Part model, mm, in its own coordinate system. A direction names the side the tool comes from. Round coordinates to 2 decimals unless told otherwise and drop trailing zeros. Write each loop counter-clockwise with the first axis right and the second up, starting at its lowest first coordinate (ties: lowest second). Pieces come first, ordered by that corner, then holes. Notation, with made-up numbers: (19, 55) -> (34, 55) arc R24 cw to (34, 88) -> close; hole circle Ø1 at (85, 25). An arc over 180 degrees is marked (long way). Return JSON: item names as keys, results as strings. Group by question number.
(1) Tool access for faces 4 (the cylindrical face through (9.139, 14.334, 64.09)), 5 (the flat face through (0, 0, -10)), 6 (the flat face through (-5, -32, 120)): list every direction of +Z, -Z, +X, -X, +Y, -Y with a clear straight run to the whole face (end or side of a thin tool).
(2) Mould opens along X. For faces 1 (the flat face through (0, 0, 0)), 2 (the flat face through (15.4, 8.4, 130)), 3 (the cylindrical face through (17.38, -33.415, 124.958)) say: +X half, -X half, draft (parallel to the pull), parting line (faces both ways), or undercut.
(3) Drill centre lines: L1, parallel to Y at x = 0, z = 95; L2, parallel to Z at x = -1.5, y = 0; L3, parallel to Y at x = -13, z = 114. Where is each one in solid material? Low to high. Write a range as from..to.
(4) Saw through at C-C (z = 49). List the corners of the cut face in (x, y).
(5) Drop flat-ended pins along their axis: pin 1 Ø1 at (x, y) = (-10, -30) entering from -Z; pin 2 Ø4 at (x, y) = (-4, 12.5) entering from +Z; pin 3 Ø4 at (y, z) = (18.5, 15) entering from -X. Give the stop position or say it passes through.
(6) Saw through at A-A (x = 0). List the corners of the cut face in (y, z).
from build123d import *

# Parameters (mm, degrees)
ESBO_O1_R                = 22
ESBO_O1_R_2              = 17
RESSALTO_EXTRUS_O1_DEPTH = 120
ESBO_O2_R                = 37.66512487
ESBO_O2_R_2              = 17
RESSALTO_EXTRUS_O2_DEPTH = 10
FILETE1_R                = 10
FILETE2_R                = 2
RESSALTO_EXTRUS_O3_START = 10
ESBO_O3_R                = 22
RESSALTO_EXTRUS_O3_DEPTH = 10


with BuildPart() as part:
    # Esboço1 → Ressalto-extrusão1 (new body)
    with BuildSketch(Plane.XY):
        Circle(ESBO_O1_R)
        Circle(ESBO_O1_R_2, mode=Mode.SUBTRACT)
    extrude(amount=RESSALTO_EXTRUS_O1_DEPTH)

    # Esboço2 → Ressalto-extrusão2 (add)
    with BuildSketch(Plane.XY.offset(120)):
        Circle(ESBO_O2_R)
        Circle(ESBO_O2_R_2, mode=Mode.SUBTRACT)
    extrude(amount=RESSALTO_EXTRUS_O2_DEPTH)

    # Filete1
    filete1_edges = [part.edges().sort_by_distance(p)[0] for p in [
        (-22, 0, 120),
    ]]
    fillet(filete1_edges, radius=FILETE1_R)

    # Filete2
    filete2_edges = [part.edges().sort_by_distance(p)[0] for p in [
        (-37.66512487, 0, 130),
        (-37.66512487, 0, 120),
    ]]
    fillet(filete2_edges, radius=FILETE2_R)

    # Esboço3 → Ressalto-extrusão3 (add)
    with BuildSketch(Plane(origin=(0, 0, 0), x_dir=(-1, 0, 0), z_dir=(0, 0, -1)).offset(RESSALTO_EXTRUS_O3_START)):
        Circle(ESBO_O3_R)
    extrude(amount=-RESSALTO_EXTRUS_O3_DEPTH)


solid = part.part
Computed values:
{
 "1": {"face 4": "+Z", "face 5": "-Z, +X, -X, +Y, -Y", "face 6": "-Z"},
 "2": {"face 1": "undercut", "face 2": "draft", "face 3": "parting line"},
 "3": {"L1": "-22..-17, 17..22", "L2": "-10..0", "L3": "-18.77..-10.95, 10.95..18.77"},
 "4": {"outline": "circle Ø44 at (0, 0); hole circle Ø34 at (0, 0)"},
 "5": {"pin 1": "z = 119.96", "pin 2": "z = 0", "pin 3": "x = -14.55"},
 "6": {"outline": "(-37.67, 122) arc R2 ccw to (-35.67, 120) -> (-32, 120) arc R10 cw to (-22, 110) -> (-22, -10) -> (22, -10) -> (22, 110) arc R10 cw to (32, 120) -> (35.67, 120) arc R2 ccw to (37.67, 122) -> (37.67, 128) arc R2 ccw to (35.67, 130) -> (17, 130) -> (17, 0) -> (-17, 0) -> (-17, 130) -> (-35.67, 130) arc R2 ccw to (-37.67, 128) -> close"}
}
